Autodesk Inventor part; units mm, degrees
ref_plane "YZ Plane" through (0, 0, 0) normal (1, 0, 0) x (0, 1, 0)
ref_plane "XZ Plane" through (0, 0, 0) normal (0, 1, 0) x (-1, 0, 0)
ref_plane "XY Plane" through (0, 0, 0) normal (0, 0, 1) x (1, 0, 0)
ref_plane "Work Plane1" through (0, 0, 0) normal (0, 0, 1) x (1, 0, 0)
sketch "Sketch1" plane through (0, 0, 0) normal (0, 0, 1) x (1, 0, 0)
  arc A0 (-11, 8.1244) -> (-11, -8.1244) centre (0, 0) ccw construction
  line L0 (-11, -8.1244) -> (-11, -24.74) construction
  line L1 (-11, -24.74) -> (11, -24.74) construction
  line L2 (11, -24.74) -> (11, -8.1244) construction
  arc A1 (11, -8.1244) -> (11, 8.1244) centre (0, 0) ccw construction
  line L3 (11, 24.74) -> (11, 8.1244) construction
  line L4 (-11, 24.74) -> (11, 24.74) construction
  line L5 (-11, 8.1244) -> (-11, 24.74) construction
  line L6 (-7.0828, 6.9741) -> (7.0828, 6.9741)
  line L7 (-7.0828, -6.9741) -> (7.0828, -6.9741)
  arc A2 (-7.0828, 6.9741) -> (-7.0828, -6.9741) centre (0, 0) ccw
  arc A3 (7.0828, -6.9741) -> (7.0828, 6.9741) centre (0, 0) ccw
  arc A4 (-3.5454, 3.44) -> (-3.5454, -3.44) centre (0, 0) ccw
  line L8 (-3.5454, 3.44) -> (-1.1656, 3.44)
  line L9 (-1.1656, 3.44) -> (-1.1656, 4.44)
  line L10 (-1.1656, 4.44) -> (-2.5, 4.44)
  line L11 (-2.5, 4.44) -> (-2.5, 5.44)
  line L12 (-2.5, 5.44) -> (2.5, 5.44)
  line L13 (2.5, 5.44) -> (2.5, 4.44)
  line L14 (2.5, 4.44) -> (1.1656, 4.44)
  line L15 (1.1656, 4.44) -> (1.1656, 3.44)
  line L16 (1.1656, 3.44) -> (3.5454, 3.44)
  arc A5 (3.5454, -3.44) -> (3.5454, 3.44) centre (0, 0) ccw
  line L17 (1.1656, -3.44) -> (3.5454, -3.44)
  line L18 (1.1656, -4.44) -> (1.1656, -3.44)
  line L19 (1.1656, -4.44) -> (2.5, -4.44)
  line L20 (2.5, -4.44) -> (2.5, -5.44)
  line L21 (2.5, -5.44) -> (-2.5, -5.44)
  line L22 (-2.5, -5.44) -> (-2.5, -4.44)
  line L23 (-1.1656, -4.44) -> (-2.5, -4.44)
  line L24 (-1.1656, -3.44) -> (-1.1656, -4.44)
  line L25 (-3.5454, -3.44) -> (-1.1656, -3.44)
  point P0 (0, 0)
extrude "Extrusion1" add sketch "Sketch1" along normal blind 2 contours L6 A3 L7 A2 | L8 L9 L10 L11 L12 L13 L14 L15 L16 A5 L17 L18 L19 L20 L21 L22 L23 L24 L25 A4
sketch "Sketch2" plane through (0, 0, 0) normal (0, 0, -1) x (-1, 0, 0)
  arc A0 (11, -8.1244) -> (11, 8.1244) centre (0, 0) ccw construction
  line L0 (11, -8.1244) -> (11, -24.74) construction
  line L1 (11, -24.74) -> (-11, -24.74) construction
  line L2 (-11, -24.74) -> (-11, -8.1244) construction
  arc A1 (-11, 8.1244) -> (-11, -8.1244) centre (0, 0) ccw construction
  line L3 (-11, 24.74) -> (-11, 8.1244) construction
  line L4 (11, 24.74) -> (-11, 24.74) construction
  line L5 (11, 8.1244) -> (11, 24.74) construction
  circle A2 centre (0, 0) radius 6.44
  circle A3 centre (0, 0) radius 4.44
  arc A4 (3.5454, -3.44) -> (3.5454, 3.44) centre (0, 0) ccw
  line L6 (3.5454, 3.44) -> (1.1656, 3.44)
  line L7 (1.1656, 3.44) -> (1.1656, 4.44)
  line L8 (1.1656, 4.44) -> (2.5, 4.44)
  line L9 (2.5, 4.44) -> (2.5, 5.44)
  line L10 (2.5, 5.44) -> (-2.5, 5.44)
  line L11 (-2.5, 5.44) -> (-2.5, 4.44)
  line L12 (-2.5, 4.44) -> (-1.1656, 4.44)
  line L13 (-1.1656, 4.44) -> (-1.1656, 3.44)
  line L14 (-1.1656, 3.44) -> (-3.5454, 3.44)
  arc A5 (-3.5454, 3.44) -> (-3.5454, -3.44) centre (0, 0) ccw
  line L15 (-1.1656, -3.44) -> (-3.5454, -3.44)
  line L16 (-1.1656, -4.44) -> (-1.1656, -3.44)
  line L17 (-1.1656, -4.44) -> (-2.5, -4.44)
  line L18 (-2.5, -4.44) -> (-2.5, -5.44)
  line L19 (-2.5, -5.44) -> (2.5, -5.44)
  line L20 (2.5, -5.44) -> (2.5, -4.44)
  line L21 (1.1656, -4.44) -> (2.5, -4.44)
  line L22 (1.1656, -3.44) -> (1.1656, -4.44)
  line L23 (3.5454, -3.44) -> (1.1656, -3.44)
  dimension "d6" = 2
extrude "Extrusion2" add sketch "Sketch2" along normal blind 8 contours A2 | A3 L6 A4 L23 | A3 L13 L12 L11 L10 L9 L8 L7 | L22 L21 L20 L19 L18 L17 L16 A3 | A3 L15 A5 L14
sketch "Sketch3" plane through (0, 0, 2) normal (0, 0, 1) x (1, 0, 0)
  arc A0 (7.0828, -6.9741) -> (7.0828, 6.9741) centre (0, 0) ccw
  circle A1 centre (0, 0) radius 2
extrude "Extrusion3" cut sketch "Sketch3" against normal through all
properties part number "ECoG_holder_cap"
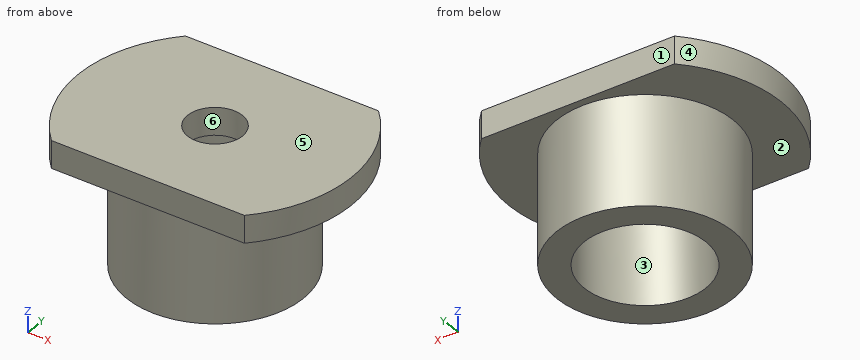
Verification items for the finished model (mm, model axes). Face numbers are marked on the shaded views. A direction names the side the tool comes from. Round coordinates to 2 decimals unless told otherwise and drop trailing zeros. Loops run counter-clockwise (first coordinate to the right, second up) from the corner with the lowest first, then second, coordinate; pieces in that order, holes last. Notation, with made-up numbers: (29, 73) - (71, 73) arc R26 cw to (71, 111) - close; hole circle Ø9 at (14.25, 63.25). An arc over 180 degrees is marked (long way). Use a Markdown table: item, result. Add a question column.
1. Section check D-D, the plane y = 2.5. Record the boundary of the cut face in (x, z).
2. Section check B-B, the plane x = 0. Record the boundary of the cut face in (y, z), plus the area to 3 significant figures.
3. Section check C-C, the plane z = 0.5. Record the boundary of the cut face in (x, y), plus the area to 3 significant figures.
4. Gauge pin test, flat ends, axial feed: pin 1 (6 mm diameter, centred on y = -1, z = -5.5, fed in from +X); pin 2 (6.5 mm diameter, centred on x = 0, y = 0, fed in from -Z). Record the tip position at first contact, or that the pin passes through.
5. Thickness scan on probe 1 along Y at (x, z) = (0, 0.6); probe 2 along Y at (x, z) = (0, -2); probe 3 along X at (y, z) = (1.5, -0.5). Record the ranges inside material, lowest first. Write a range as [from, to].
6. Section check A-A, the plane y = 0. Record the boundary of the cut face in (x, z), plus the area to 3 significant figures.
7. Access from +Z, -Z, +X, -X, +Y, -Y to the whole of each face (thin tool, end or side, straight path). Record for the marked faces 1 and 2.
8. Release check for a two-part mould opening along X. For the marked faces 3, 4, 5 and 6 record: released by +X, released by -X, zero draft, split by the parting line, or undercut.
Checks:
| question | item | result |
|---|---|---|
| 1 | outline | (-9.62, 0) - (-5.93, 0) - (-5.93, -8) - (-3.67, -8) - (-3.67, 0) - (3.67, 0) - (3.67, -8) - (5.93, -8) - (5.93, 0) - (9.62, 0) - (9.62, 2) - (-9.62, 2) - close |
| 2 | outline | (-6.97, 0) - (-6.44, 0) - (-6.44, -8) - (-4.44, -8) - (-4.44, 0) - (-2, 0) - (-2, 2) - (-6.97, 2) - close; (2, 0) - (4.44, 0) - (4.44, -8) - (6.44, -8) - (6.44, 0) - (6.97, 0) - (6.97, 2) - (2, 2) - close |
| 2 | area | 51.9 mm^2 |
| 3 | outline | (-7.08, -6.97) - (7.08, -6.97) arc R9.94 ccw to (7.08, 6.97) - (-7.08, 6.97) arc R9.94 ccw to start; hole circle Ø4 at (0, 0) |
| 3 | area | 240 mm^2 |
| 4 | pin 1 | stops at x = 6.44 |
| 4 | pin 2 | stops at z = 0 |
| 5 | probe 1 | y = [-6.97, -2], [2, 6.97] |
| 5 | probe 2 | y = [-6.44, -4.44], [4.44, 6.44] |
| 5 | probe 3 | x = [-6.26, -4.18], [4.18, 6.26] |
| 6 | outline | (-9.94, 0) - (-6.44, 0) - (-6.44, -8) - (-4.44, -8) - (-4.44, 0) - (-2, 0) - (-2, 2) - (-9.94, 2) - close; (2, 0) - (4.44, 0) - (4.44, -8) - (6.44, -8) - (6.44, 0) - (9.94, 0) - (9.94, 2) - (2, 2) - close |
| 6 | area | 63.8 mm^2 |
| 7 | face 1 | +Z, -Z, +X, -X, +Y |
| 7 | face 2 | -Z |
| 8 | face 3 | undercut |
| 8 | face 4 | released by -X |
| 8 | face 5 | zero draft |
| 8 | face 6 | undercut |
